The listing builds one solid part. Answer for the finished solid, in the listing's coordinates (mm). A direction names the side the tool comes from. Coordinates: 2 decimals unless noted, no trailing zeros. Loops run counter-clockwise (first coordinate to the right, second up) from the corner with the lowest first, then second, coordinate; pieces in that order, holes last. Notation, with made-up numbers: M 2.25,37.5 L 35.25,37.5 A15 ccw 35.25,45.5 Z; hole C 33.25,42 d5. An arc over 180 degrees is marked long. Return JSON: item names as keys, results as strings. Group by question number.
1. Straight lines are drawn through the part: L1, parallel to Z at x = -88, y = -1; L2, parallel to X at y = 19, z = 97.5. For each, find the intervals that lie inside material, in ascending order. Write a range as from..to.
2. The mould has two halves that part along X. Classify faces 1 (the face through (-3, -1, 133.35)), 2 (the face through (245.237, -1, -2)), 3 (the face through (-245.237, -1, -2)), 4 (the face through (-3, 1, 146.05)): pulls with the +X half, pulls with the -X half, needs draft (parallel to the pull), parting line crosses it, or undercut.
3. Section A-A (z = -113) is taken. Write down the section's boundary in (x, y) (3 decimals), then the cut area to 3 significant figures.
4. Section B-B (x = 154) is taken. Write down the section's boundary in (y, z), then the cut area to 3 significant figures.
5. Section C-C (y = 13.5) is taken. Write down the section's boundary in (x, z).
6. Given P1, Ø1.5, axis at x = 83, y = 8, coming from the -Z side, flat-ended and moving along its own axis, determine where the tip first touches the part or whether it passes through.
7. Which of the six approach directions +Z, -Z, +X, -X, +Y, -Y give full straight-line access (tool end or side, diameter ignored) to faces 5 (the face through (232.537, -1, -2)), 6 (the face through (-19, -38.1, -140))?
```python
from build123d import *

# Parameters (mm, degrees)
F0_W     = 490.474
F0_H     = 292.1
F0_W_2   = 465.074
F0_H_2   = 266.7
F1_DEPTH = 38.1
F2_R     = 3.175
F3_DEPTH = 292.354


with BuildPart() as f1:
    # F0 (on Front) → F1 (new body, symmetric)
    with BuildSketch(Plane.XZ):
        Rectangle(F0_W, F0_H)
        Rectangle(F0_W_2, F0_H_2, mode=Mode.SUBTRACT)
    extrude(amount=F1_DEPTH, both=True)

    # F2 (on face) → F3 (join)
    with BuildSketch(Plane.XY.offset(146.05)):
        with Locations((-207.137, 0)):
            Circle(F2_R)
    extrude(amount=-F3_DEPTH)


solid = f1.part
```
Worked out:
{
 "1": {"L1": "-146.05..-133.35, 133.35..146.05", "L2": "-245.24..-232.54, 232.54..245.24"},
 "2": {"face 1": "undercut", "face 2": "pulls with the +X half", "face 3": "pulls with the -X half", "face 4": "needs draft"},
 "3": {"outline": "M -245.237,-38.1 L -232.537,-38.1 L -232.537,38.1 L -245.237,38.1 Z; C -207.137,0 d6.35; M 232.537,-38.1 L 245.237,-38.1 L 245.237,38.1 L 232.537,38.1 Z", "area": "1,970 mm^2"},
 "4": {"outline": "M -38.1,-146.05 L 38.1,-146.05 L 38.1,-133.35 L -38.1,-133.35 Z; M -38.1,133.35 L 38.1,133.35 L 38.1,146.05 L -38.1,146.05 Z", "area": "1,940 mm^2"},
 "5": {"outline": "M -245.24,-146.05 L 245.24,-146.05 L 245.24,146.05 L -245.24,146.05 Z; hole M -232.54,-133.35 L 232.54,-133.35 L 232.54,133.35 L -232.54,133.35 Z"},
 "6": {"P1": "z = -146.05"},
 "7": {"face 5": "+Y, -Y", "face 6": "+Z, -Z, +X, -X, -Y"}
}
